Source: three-view drawing plus pictorial views. Frame: mm from the lowest corner of the part. Round coordinates to 2 decimals unless told otherwise and drop trailing zeros. Order: outer loops, then holes, each group sorted by start corner. A loop starts at its lowest first (then second) coordinate and runs counter-clockwise, first axis right, second up. Notation, with made-up numbers: M 68.25,40 L 95.25,40 A22 cw 95.25,57 Z; hole C -32.75,-28 d10. An arc over 180 degrees is marked long. Return JSON: item names as keys, results as strings. Group by question number.
Q1. Cut plane A-A on y = 92.16. Output: boundary loops of the cut face in (x, z).
Q2. Cut plane B-B on z = 0.3. Count the separate pieces of the cut face and the enclosed holes in it, and give its area (3 significant figures).
Q3. Ray query, probe 1 along X at (y, z) = (42.71, 0.4); probe 2 along Y at (x, z) = (10.25, 0.6); probe 3 along Y at (x, z) = (7.5, 1.1). Return the intervals inside material, ascending.
Q4. Contact query for flat-ended pins moving along their axis: pin 1 (0.6 mm diameter, centred on y = 50.5, z = 0.5, fed in from +X); pin 2 (0.6 mm diameter, centred on y = 79.5, z = 0.5, fed in from -X). Output: stop coordinate, or through.
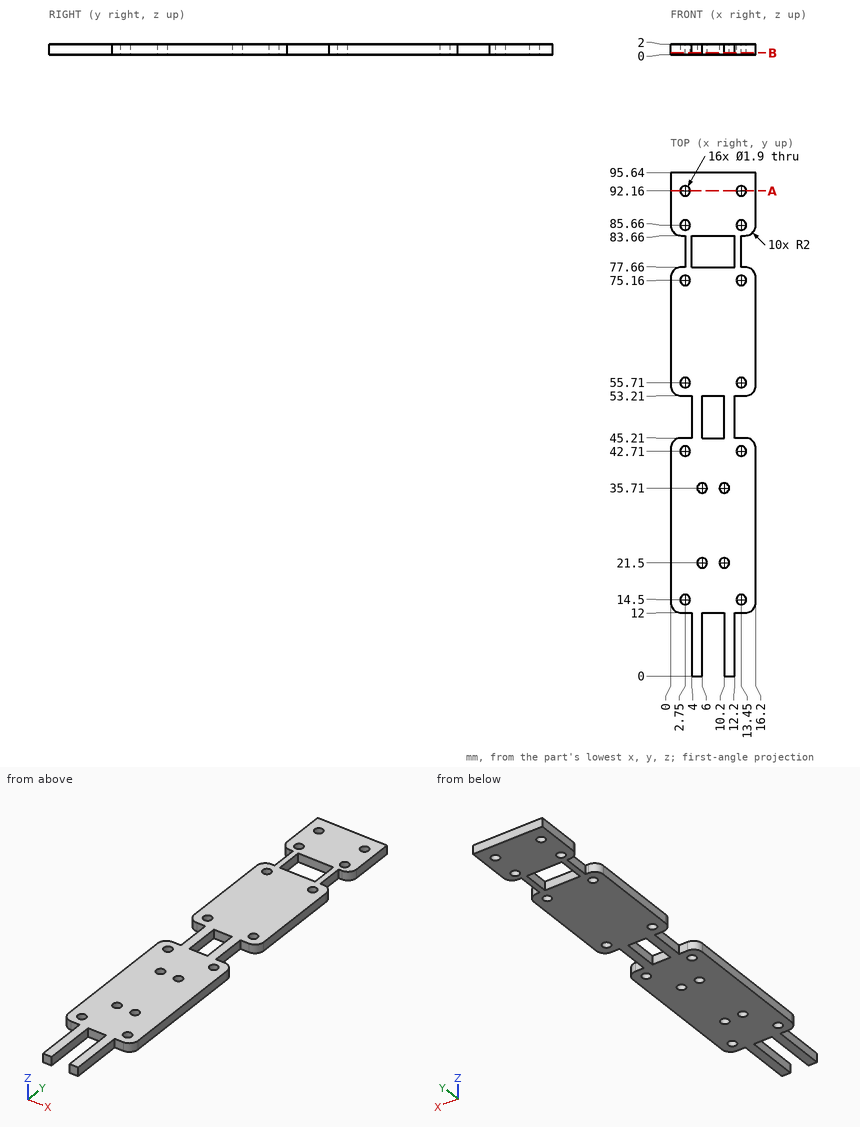
Result sheet:
{
 "1": {"outline": "M 0,0 L 1.8,0 L 1.8,2 L 0,2 Z; M 3.7,0 L 12.5,0 L 12.5,2 L 3.7,2 Z; M 14.4,0 L 16.2,0 L 16.2,2 L 14.4,2 Z"},
 "2": {"separate pieces": "1", "enclosed holes": "18", "area": "1,170 mm²"},
 "3": {"probe 1": "x = 0 to 1.8, 3.7 to 12.5, 14.4 to 16.2", "probe 2": "y = 0 to 20.55, 22.45 to 34.76, 36.66 to 77.66, 83.66 to 95.64", "probe 3": "y = 12 to 45.21, 53.21 to 77.66, 83.66 to 95.64"},
 "4": {"pin 1": "stops at x = 12.2", "pin 2": "stops at x = 2.75"}
}
